Geometry check sheet. Reference: the model listing, model coordinates, mm. Face numbers are marked on the shaded views. A direction names the side the tool comes from. Give positions to 0.01 mm unless a question says otherwise; leave off trailing zeros. Loops run counter-clockwise (first coordinate to the right, second up) from the corner with the lowest first, then second, coordinate; pieces in that order, holes last. Notation, with made-up numbers: (-9.75, -20.5) - (-2.75, -20.5) arc R15 cw to (-2.75, 3.5) - close; hole circle Ø2 at (52.25, 53). An arc over 180 degrees is marked (long way). Use a Markdown table: item, result. Add a question column.
1. Cross-section at B-B on x = -0.95. Enter the section's corners in (y, z).
2. Set-up check for the marked faces 1 and 2: record each of +Z, -Z, +X, -X, +Y, -Y from which the full face is reachable in a straight line by a thin tool's end or side.
3. Cross-section at A-A on z = 0. Enter the section's corners in (x, y).
4. Draft check along Z on the marked faces 3, 4 and 5. Enter one of: pulls with the +Z half, pulls with the -Z half, needs draft (parallel to the pull), parting line crosses it, or undercut.
5. Depth check by flat-ended pin: P1, Ø1.3, axis at x = 0, z = -0.5, coming from the +Y side; P2, Ø1, axis at x = 0, y = 2.5, coming from the -Z side; P3, Ø1.2, axis at x = -0.5, z = -0.5, coming from the -Y side; P4, Ø1, axis at y = 2.5, z = -0.5, coming from the -X side. Enter the tip coordinate at first touch or a pass-through.
6. Cross-section at C-C on y = 6.5. Enter the section's corners in (x, z), and give its area (3 significant figures).
7. Material ranges on L1, parallel to Y at x = -1.2, z = -0.65; L2, parallel to Z at x = -0.8, y = 17.5; L3, parallel to Z at x = -0.65, y = 18, recorded low to high.
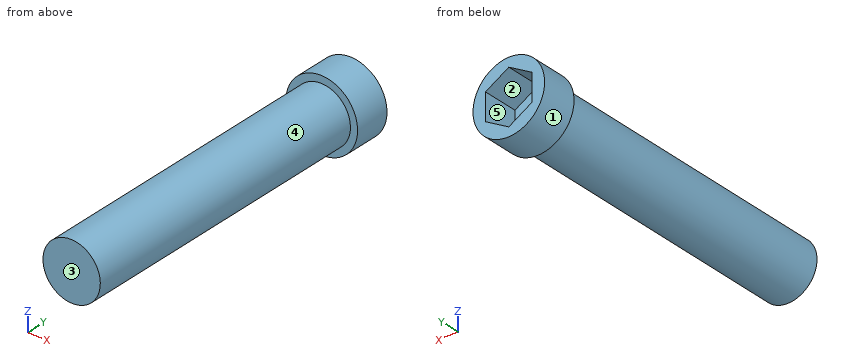
from build123d import *

# Parameters (mm, degrees)
SKETCH1_R    = 1.6
LENGTH_DEPTH = 17
SKETCH2_R    = 2
CAP_DEPTH    = 2
HEX_2_DEPTH  = 2


with BuildPart() as part:
    # Sketch1 → Length (new body)
    with BuildSketch(Plane(origin=(0, 0, 0), x_dir=(1, 0, 0), z_dir=(0, 1, 0))):
        with Locations(Location((0, 0, 0), (0, 0, 270))):
            Circle(SKETCH1_R)
    extrude(amount=LENGTH_DEPTH)

    # Sketch2 → Cap (add)
    with BuildSketch(Plane(origin=(0, 17, 0), x_dir=(1, 0, 0), z_dir=(0, 1, 0))):
        with Locations(Location((0, 0, 0), (0, 0, 270))):
            Circle(SKETCH2_R)
    extrude(amount=CAP_DEPTH)

    # Sketch3 → Hex 2 (cut)
    with BuildSketch(Plane(origin=(0, 19, 0), x_dir=(1, 0, 0), z_dir=(0, 1, 0))):
        Polygon((0, 1.5), (-1.299038106, 0.75), (-1.299038106, -0.75), (0, -1.5), (1.299038106, -0.75), (1.299038106, 0.75), align=None)
    extrude(amount=-HEX_2_DEPTH, mode=Mode.SUBTRACT)


solid = part.part
Values found:
| question | item | result |
|---|---|---|
| 1 | outline | (0, -1.29) - (17, -1.29) - (17, -1.76) - (19, -1.76) - (19, -0.95) - (17, -0.95) - (17, 0.95) - (19, 0.95) - (19, 1.76) - (17, 1.76) - (17, 1.29) - (0, 1.29) - close |
| 2 | face 1 | +Y, -Y |
| 2 | face 2 | +Y |
| 3 | outline | (-2, 17) - (-1.6, 17) - (-1.6, 0) - (1.6, 0) - (1.6, 17) - (2, 17) - (2, 19) - (1.3, 19) - (1.3, 17) - (-1.3, 17) - (-1.3, 19) - (-2, 19) - close |
| 4 | face 3 | needs draft |
| 4 | face 4 | parting line crosses it |
| 4 | face 5 | undercut |
| 5 | P1 | stops at y = 17 |
| 5 | P2 | stops at z = -1.6 |
| 5 | P3 | stops at y = 0 |
| 5 | P4 | stops at x = -1.6 |
| 6 | outline | circle Ø3.2 at (0, 0) |
| 6 | area | 8.04 mm2 |
| 7 | L1 | y = 0 to 17 |
| 7 | L2 | z = -1.83 to -1.04, 1.04 to 1.83 |
| 7 | L3 | z = -1.89 to -1.12, 1.12 to 1.89 |
